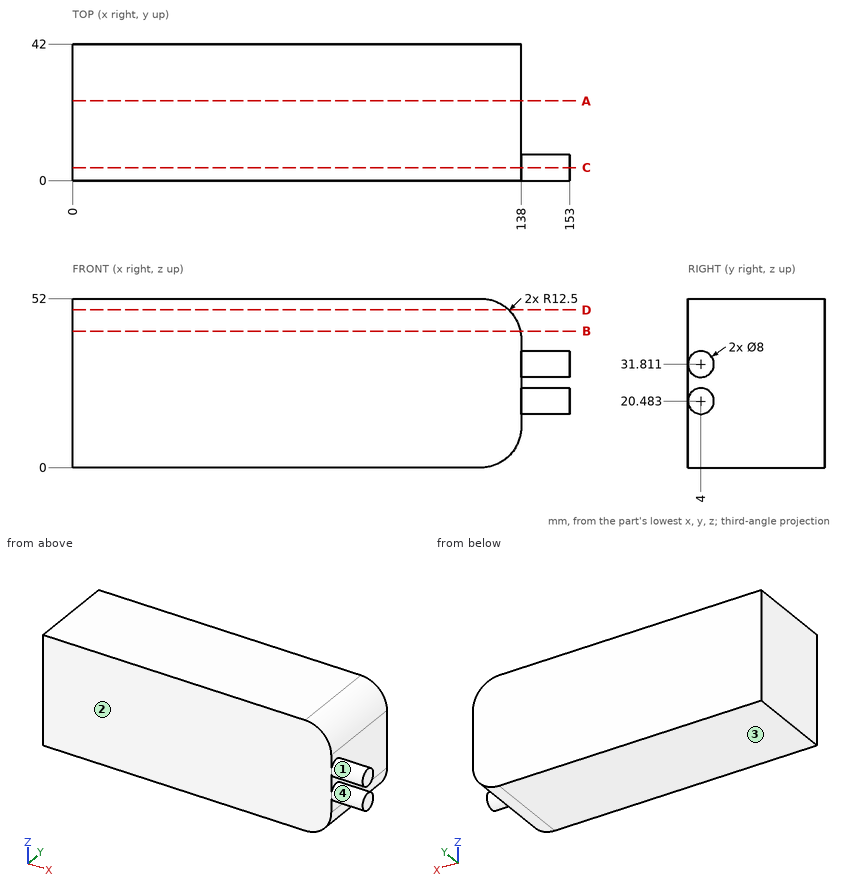
Print and shaded views of the part. All mm, measured from the part's lowest x, y and z. Give positions to 0.01 mm unless a question says otherwise; leave off trailing zeros. Order: outer loops, then holes, each group sorted by start corner. A loop starts at its lowest first (then second) coordinate and runs counter-clockwise, first axis right, second up. Notation, with made-up numbers: (89, 6.25) - (130, 6.25) arc R8 ccw to (130, 18.25) - close; hole circle Ø7 at (25.25, 74). An arc over 180 degrees is marked (long way). One line per item, written item: value.
Item 1: Two-plate mould, pull along Z, no slides. Class the marked faces 1, 2, 3 and 4: released by +Z, released by -Z, zero draft, split by the parting line, or undercut.
Response values:
face 1: undercut
face 2: zero draft
face 3: released by -Z
face 4: undercut
Item 2: Slice it at A-A (y = 24.5). List the corners of the cut face in (x, z).
Response values:
outline: (0, 0) - (125.5, 0) arc R12.5 ccw to (138, 12.5) - (138, 39.5) arc R12.5 ccw to (125.5, 52) - (0, 52) - close
Item 3: Slice it at D-D (z = 48.5). List the corners of the cut face in (x, y) (1 decimal), then the cut area to 3 significant figures.
Response values:
outline: (0, 0) - (134.2, 0) - (134.2, 42) - (0, 42) - close
area: 5,640 mm2
Item 4: Pin check, flat tip, straight feed: pin 1 Ø1 at (y, z) = (9, 40.5) entering from +X. Stop position of the tip, or through.
Response values:
pin 1: x = 137.99
Item 5: Wall check: line 1 (X direction, y = 26, z = 26); line 2 (Y direction, x = 146, z = 20.5); line 3 (X direction, y = 25.5, z = 47). Give the ranges that are in metal, low to high.
Response values:
line 1: 0 to 138
line 2: 0 to 8
line 3: 0 to 135.5
Item 6: Slice it at B-B (z = 42). List the corners of the cut face in (x, y).
Response values:
outline: (0, 0) - (137.75, 0) - (137.75, 42) - (0, 42) - close
Item 7: Slice it at C-C (y = 4). List the corners of the cut face in (x, z), then the cut area to 3 significant figures.
Response values:
outline: (0, 0) - (125.5, 0) arc R12.5 ccw to (138, 12.5) - (138, 16.48) - (153, 16.48) - (153, 24.48) - (138, 24.48) - (138, 27.81) - (153, 27.81) - (153, 35.81) - (138, 35.81) - (138, 39.5) arc R12.5 ccw to (125.5, 52) - (0, 52) - close
area: 7,350 mm2
